Source: CAD feature listing. Evaluate the final solid. Frame: model axes, mm. Give positions to 0.01 mm unless a question says otherwise; leave off trailing zeros. Write each loop counter-clockwise with the first axis right and the second up, starting at its lowest first coordinate (ties: lowest second). Pieces come first, ordered by that corner, then holes. Notation, with made-up numbers: (17, 42) - (32, 42) arc R20 ccw to (32, 76) - close; hole circle Ø6 at (59, -11). An arc over 180 degrees is marked (long way). One line per question, with ' | ' between items. Start each with the question number.
(1) Ray query, line 1 (Z direction, x = 5, y = -9.35); line 2 (X direction, y = -9.45, z = 488.33); line 3 (X direction, y = -1.5, z = 98.5). Return the intervals inside material, ascending. Write a range as [from, to].
(2) Pin query (flat end, axial travel): pin 1 (5 mm diameter, centred on x = 5, z = 488.33, fed in from -Y). Return the tip coordinate at first contact, or that it passes through.
(3) Section B-B, the plane z = 370. Return loops of the section in (x, y).
(4) Section A-A, the plane y = -1.75. Return loops of the section in (x, z).
```python
from build123d import *

# Parameters (mm, degrees)
SKETCH_1_W                = 20
SKETCH_1_H                = 20
SKETCH_1_W_2              = 18
SKETCH_1_H_2              = 18
EXTRUDE_1_DEPTH           = 493.33
SKETCH_5_R                = 2
CUT_EXTRUDE_12_DEPTH      = 20
SKETCH_6_R                = 2
CUT_EXTRUDE_13_DEPTH      = 146
CUT_EXTRUDE_13_DEPTH_BACK = 84


with BuildPart() as part:
    # Sketch 1 → Extrude 1 (new body)
    with BuildSketch(Plane.XY):
        Rectangle(SKETCH_1_W, SKETCH_1_H)
        Rectangle(SKETCH_1_W_2, SKETCH_1_H_2, mode=Mode.SUBTRACT)
    extrude(amount=EXTRUDE_1_DEPTH)

    # Sketch 5 → Cut-Extrude 12 (cut)
    with BuildSketch(Plane.XZ.offset(-9)):
        with Locations((-5, 9)):
            Circle(SKETCH_5_R)
        with Locations((5, 9)):
            Circle(SKETCH_5_R)
    extrude(amount=-CUT_EXTRUDE_12_DEPTH, mode=Mode.SUBTRACT)

    # Sketch 6 → Cut-Extrude 13 (cut, two sides)
    with BuildSketch(Plane(origin=(0, -9, 0), x_dir=(1, 0, 0), z_dir=(0, 1, 0))) as cut_extrude_13_sk:
        with Locations((303.56, -9)):
            Circle(SKETCH_6_R)
        with Locations((5, -9)):
            Circle(SKETCH_6_R)
        with Locations((-5, -9)):
            Circle(SKETCH_6_R)
        with Locations((15.394157217, -478.33)):
            Circle(SKETCH_6_R)
        with Locations((15.394157217, -488.33)):
            Circle(SKETCH_6_R)
        with Locations((5, -488.33)):
            Circle(SKETCH_6_R)
        with Locations((-5, -488.33)):
            Circle(SKETCH_6_R)
        with Locations((283.56, -488.33)):
            Circle(SKETCH_6_R)
        with Locations((283.56, -478.33)):
            Circle(SKETCH_6_R)
        with Locations((293.56, -488.33)):
            Circle(SKETCH_6_R)
        with Locations((303.56, -488.33)):
            Circle(SKETCH_6_R)
        with Locations((293.56, -9)):
            Circle(SKETCH_6_R)
    extrude(amount=CUT_EXTRUDE_13_DEPTH, mode=Mode.SUBTRACT)
    extrude(cut_extrude_13_sk.sketch, amount=-CUT_EXTRUDE_13_DEPTH_BACK, mode=Mode.SUBTRACT)


solid = part.part
```
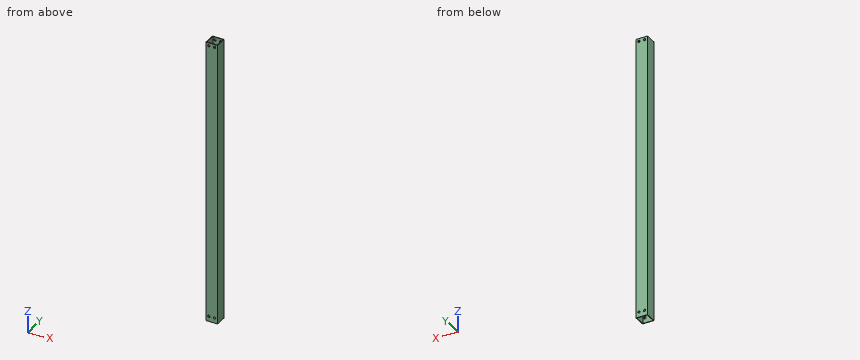
Check sheet entries:
1) line 1: [0, 7], [11, 486.33], [490.33, 493.33] | line 2: [-10, -7], [-3, 3], [7, 10] | line 3: [-10, -9], [9, 10]
2) pin 1: y = -10
3) outline: (-10, -10) - (10, -10) - (10, 10) - (-10, 10) - close; hole (-9, -9) - (9, -9) - (9, 9) - (-9, 9) - close
4) outline: (-10, 0) - (-9, 0) - (-9, 493.33) - (-10, 493.33) - close; (9, 0) - (10, 0) - (10, 493.33) - (9, 493.33) - close
